Check sheet for the modelled part. Datum: model origin and axes. Units: mm. A direction names the side the tool comes from. Round coordinates to 2 decimals unless told otherwise and drop trailing zeros. Order: outer loops, then holes, each group sorted by start corner. A loop starts at its lowest first (then second) coordinate and runs counter-clockwise, first axis right, second up.
```python
from build123d import *

# Parameters (mm, degrees)
F0_W     = 80
F0_H     = 50
F1_DEPTH = 45
F2_R     = 5
F3_T     = -2.5


with BuildPart() as f1:
    # F0 (on Top) → F1 (new body)
    with BuildSketch(Plane.XY):
        with Locations((6.780662, 7.407585)):
            Rectangle(F0_W, F0_H)
    extrude(amount=F1_DEPTH)

    # F2
    f2_edges = [f1.edges().sort_by_distance(p)[0] for p in [
        (-33.219338, -17.592415, 22.5),
        (46.780662, -17.592415, 22.5),
        (46.780662, 32.407585, 22.5),
        (-33.219338, 32.407585, 22.5),
        (46.780662, 7.407585, 0),
        (6.780662, 32.407585, 0),
        (-33.219338, 7.407585, 0),
        (6.780662, -17.592415, 0),
    ]]
    fillet(f2_edges, radius=F2_R)

    # F3
    f3_openings = [f1.faces().sort_by_distance(p)[0] for p in [
        (6.780662, 7.407585, 45),
    ]]
    offset(amount=F3_T, openings=f3_openings)


solid = f1.part
```
Item 1: Go/stop test with a flat-tipped pin: P1, Ø12, axis at x = 17, y = 0.5, coming from the +Z side. Record where the tip stops, or that it passes through.
Answer:
P1: stops at z = 2.5
Item 2: Sectioned sample at B-B (x = -18). Record the cut outline in (y, z).
Answer:
outline: (-17.59, 5) arc R5 ccw to (-12.59, 0) - (27.41, 0) arc R5 ccw to (32.41, 5) - (32.41, 45) - (29.91, 45) - (29.91, 5) arc R2.5 cw to (27.41, 2.5) - (-12.59, 2.5) arc R2.5 cw to (-15.09, 5) - (-15.09, 45) - (-17.59, 45) - close
Item 3: Access from +Z, -Z, +X, -X, +Y, -Y to the whole of each face (thin tool, end or side, straight path). Record for faces 4 (the cylindrical face through (43.53, -14.38, 25.28)), 5 (the cylindrical face through (7.271, -16.167, 1.504)).
Answer:
face 4: +Z
face 5: -Z, +X, -X, -Y
Item 4: Release check for a two-part mould opening along Y. For faces 1 (the cylindrical face through (-30.006, 7.688, 3.252)), 2 (the cylindrical face through (-31.79, -16.09, 25.28)), 3 (the cylindrical face through (7.27, 30.98, 1.5)) record: released by +Y, released by -Y, zero draft, split by the parting line, or undercut.
Answer:
face 1: undercut
face 2: released by -Y
face 3: released by +Y
Item 5: Sectioned sample at C-C (y = 22.5). Record the cut outline in (x, z), and give its area (3 significant figures).
Answer:
outline: (-33.22, 5) arc R5 ccw to (-28.22, 0) - (41.78, 0) arc R5 ccw to (46.78, 5) - (46.78, 45) - (44.28, 45) - (44.28, 5) arc R2.5 cw to (41.78, 2.5) - (-28.22, 2.5) arc R2.5 cw to (-30.72, 5) - (-30.72, 45) - (-33.22, 45) - close
area: 404 mm2
Item 6: Scan lines: line 1 along X through (y, z) = (0, 11); line 2 along Y through (x, z) = (1, 27.5); line 3 along Z through (x, y) = (23.5, 15.5). Record each from-to range of solid material in increasing order.
Answer:
line 1: x = -33.22 to -30.72, 44.28 to 46.78
line 2: y = -17.59 to -15.09, 29.91 to 32.41
line 3: z = 0 to 2.5
Item 7: Sectioned sample at A-A (z = 12.5). Record the cut outline in (x, y).
Answer:
outline: (-33.22, -12.59) arc R5 ccw to (-28.22, -17.59) - (41.78, -17.59) arc R5 ccw to (46.78, -12.59) - (46.78, 27.41) arc R5 ccw to (41.78, 32.41) - (-28.22, 32.41) arc R5 ccw to (-33.22, 27.41) - close; hole (-30.72, -12.59) arc R2.5 ccw to (-28.22, -15.09) - (41.78, -15.09) arc R2.5 ccw to (44.28, -12.59) - (44.28, 27.41) arc R2.5 ccw to (41.78, 29.91) - (-28.22, 29.91) arc R2.5 ccw to (-30.72, 27.41) - close
